Answer from the drawing. Dimensions are ordinates in mm from the lowest x, y and z of the part. Give positions to 0.01 mm unless a question says otherwise; leave off trailing zeros. Loops run counter-clockwise (first coordinate to the right, second up) from the corner with the lowest first, then second, coordinate; pieces in that order, holes last. Notation, with made-up numbers: (-36.5, 15) - (-13.5, 15) arc R25 cw to (-13.5, 43) - close; hole circle Ø1 at (39, 63). An arc over 180 degrees is marked (long way). One line per item, written item: value.
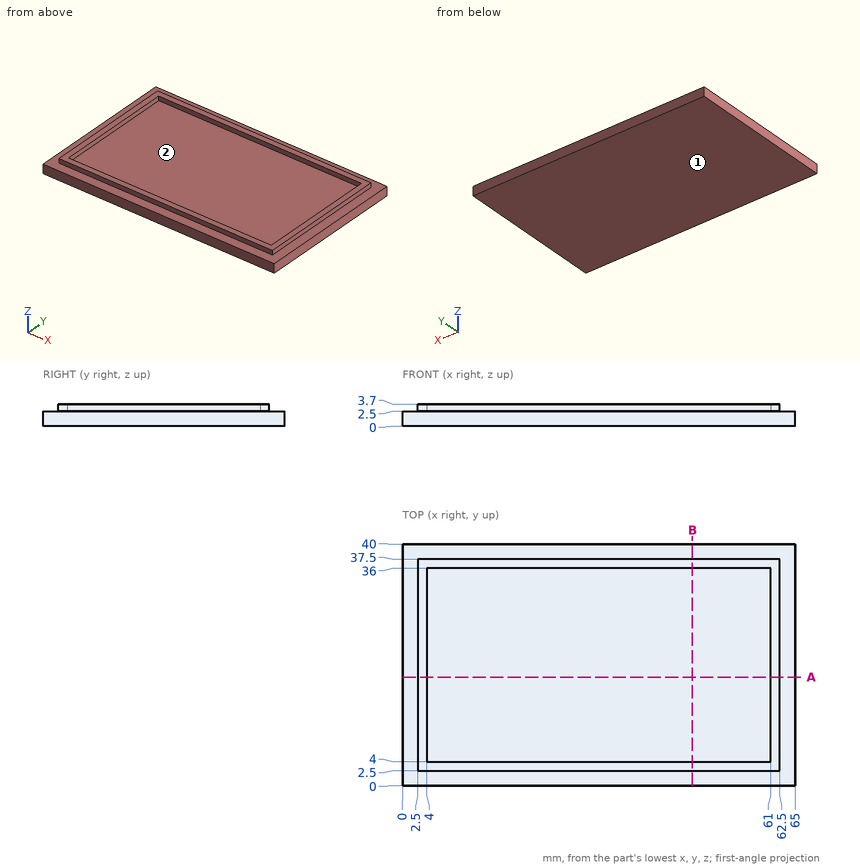
1. Flat-ended cylindrical pins translate along their axes: pin 1 Ø0.6 at (x, z) = (41.5, 3) entering from +Y; pin 2 Ø1 at (y, z) = (28, 3.5) entering from -X; pin 3 Ø0.6 at (x, z) = (23.5, 3.5) entering from -Y. Find the tip coordinate at first contact, or state that the pin passes through.
Output:
pin 1: stops at y = 37.5
pin 2: stops at x = 2.5
pin 3: stops at y = 2.5
2. Section B-B (x = 48) is taken. Write down the section's boundary in (y, z), and give its area (3 significant figures).
Output:
outline: (0, 0) - (40, 0) - (40, 2.5) - (37.5, 2.5) - (37.5, 3.7) - (36, 3.7) - (36, 2.5) - (4, 2.5) - (4, 3.7) - (2.5, 3.7) - (2.5, 2.5) - (0, 2.5) - close
area: 104 mm²
3. The mould has two halves that part along Y. Classify the marked faces 1 and 2: released by +Y, released by -Y, zero draft, split by the parting line, or undercut.
Output:
face 1: zero draft
face 2: undercut
4. Find the intervals of material crossed by line 1 along Y through (x, z) = (6, 2.75); line 2 along X through (y, z) = (34, 2.9); line 3 along Z through (x, y) = (6.5, 13.5), in increasing order.
Output:
line 1: y = 2.5 to 4, 36 to 37.5
line 2: x = 2.5 to 4, 61 to 62.5
line 3: z = 0 to 2.5
5. Section A-A (y = 18) is taken. Write down the section's boundary in (x, z), and give its area (3 significant figures).
Output:
outline: (0, 0) - (65, 0) - (65, 2.5) - (62.5, 2.5) - (62.5, 3.7) - (61, 3.7) - (61, 2.5) - (4, 2.5) - (4, 3.7) - (2.5, 3.7) - (2.5, 2.5) - (0, 2.5) - close
area: 166 mm²
